Input: part model. Units: mm. Frame: model coordinates. A direction names the side the tool comes from. Coordinates: 2 decimals unless noted, no trailing zeros. Write each loop counter-clockwise with the first axis right and the second up, starting at its lowest first coordinate (ties: lowest second). Pieces come first, ordered by that corner, then holes. Notation, with made-up numbers: (75.5, 22) - (96.5, 22) arc R24 ccw to (96.5, 54) - close; hole circle Ø1 at (79, 14.25). An arc over 180 degrees is marked (long way). Put each result on its own line as item: value. Start each with the question number.
1. Line query: line 1 (Z direction, x = 0.5, y = 54); line 2 (Y direction, x = 5.5, z = 31.5); line 3 (Y direction, x = -42, z = 17). Output: solid intervals per line, ascending.
2. Cut plane D-D, the plane z = 22.5. Return loops of the section in (x, y), and give its area (3 significant figures).
3. Access query for faces 1 (the flat face through (-25.67, -70.96, 19.14)), 2 (the flat face through (31.75, -16, 16)), 3 (the flat face through (-9, 0, 25.4)), 4 (the flat face through (-6.35, 62, 38)). Directions: +Z, -Z, +X, -X, +Y, -Y. A direction counts if a zero-diameter tool reaches every point of the face in a straight line with its end or side. Return the directions, or none.
4. Pull-direction query (Y, two-part tool) for faces 5 (the cylindrical face through (-5.728, -79.117, 4.539)), 6 (the flat face through (8.733, 71.285, 21.785)), 7 (the flat face through (-40.73, -16.73, 19.14)); classes: released by +Y, released by -Y, zero draft, split by the parting line, or undercut.
5. Cut plane A-A, the plane z = 30. Return loops of the section in (x, y), and give its area (3 significant figures).
6. Pin query (flat end, axial travel): pin 1 (12 mm diameter, centred on y = -2.5, z = 30, fed in from +X); pin 2 (2 mm diameter, centred on x = 29, y = -61, fed in from +Z); pin 3 (6 mm diameter, centred on x = 26, z = 26, fed in from +Y). Return the tip coordinate at first contact, or that it passes through.
from build123d import *

# Parameters (mm, degrees)
F0_W        = 88.9
F0_H        = 165.1
F1_DEPTH    = 6.35
F2_DEPTH    = 25.4
F3_DEPTH    = 50.8
F4_R        = 6.34999
F5_C1_SIZE2 = 12.7
F5_C1_SIZE  = 7.3323484187
F5_C2_SIZE2 = 12.7
F5_C2_SIZE  = 7.3323484187
F5_C3_SIZE2 = 12.7
F5_C3_SIZE  = 7.3323484187
F5_C4_SIZE2 = 12.7
F5_C4_SIZE  = 7.3323484187
F5_C5_SIZE2 = 7.3323484187
F5_C5_SIZE  = 12.7
F5_C6_SIZE2 = 7.3323484187
F5_C6_SIZE  = 12.7
F5_C7_SIZE2 = 12.7
F5_C7_SIZE  = 7.3323484187
F5_C8_SIZE2 = 7.3323484187
F5_C8_SIZE  = 12.7


# Not quite as in the source:
# - a fillet or chamfer is up to 0.001 mm smaller than in the source, because OpenCascade refuses the exact size


with BuildPart() as f1:
    # F0 (on Top) → F1 (new body)
    with BuildSketch(Plane.XY):
        with Locations((-6.35, 1.5239301443)):
            Rectangle(F0_W, F0_H)
        Polygon((-44.45, 39.6239301443), (-44.45, 77.7239301443), (-6.35, 77.7239301443), (31.75, 77.7239301443), (31.75, -36.5760698557), (31.75, -74.6760698557), (-6.35, -74.6760698557), (-44.45, -74.6760698557), align=None, mode=Mode.SUBTRACT)
        with BuildLine():
            Line((31.75, 77.7239301443), (-6.35, 77.7239301443))
            Line((-6.35, 77.7239301443), (-6.35, 45.9739301443))
            ThreePointArc((-6.35, 45.9739301443), (-8.2098719395, 41.4838020838), (-12.7, 39.6239301443))
            Line((-12.7, 39.6239301443), (-44.45, 39.6239301443))
            Line((-44.45, 39.6239301443), (-44.45, -74.6760698557))
            Line((-44.45, -74.6760698557), (-6.35, -74.6760698557))
            Line((-6.35, -74.6760698557), (-6.35, -42.9260698557))
            ThreePointArc((-6.35, -42.9260698557), (-4.4901280605, -38.4359417952), (0, -36.5760698557))
            Line((0, -36.5760698557), (31.75, -36.5760698557))
            Line((31.75, -36.5760698557), (31.75, 77.7239301443))
        make_face()
        with BuildLine():
            Line((-6.35, 77.7239301443), (-44.45, 77.7239301443))
            Line((-44.45, 77.7239301443), (-44.45, 39.6239301443))
            Line((-44.45, 39.6239301443), (-12.7, 39.6239301443))
            ThreePointArc((-12.7, 39.6239301443), (-8.2098719395, 41.4838020838), (-6.35, 45.9739301443))
            Line((-6.35, 45.9739301443), (-6.35, 77.7239301443))
        make_face()
        with BuildLine():
            Line((31.75, -74.6760698557), (31.75, -36.5760698557))
            Line((31.75, -36.5760698557), (0, -36.5760698557))
            ThreePointArc((0, -36.5760698557), (-4.4901280605, -38.4359417952), (-6.35, -42.9260698557))
            Line((-6.35, -42.9260698557), (-6.35, -74.6760698557))
            Line((-6.35, -74.6760698557), (31.75, -74.6760698557))
        make_face()
    extrude(amount=F1_DEPTH)

    # F0 (on Top) → F2 (join)
    with BuildSketch(Plane.XY):
        with BuildLine():
            Line((31.75, 77.7239301443), (-6.35, 77.7239301443))
            Line((-6.35, 77.7239301443), (-6.35, 45.9739301443))
            ThreePointArc((-6.35, 45.9739301443), (-8.2098719395, 41.4838020838), (-12.7, 39.6239301443))
            Line((-12.7, 39.6239301443), (-44.45, 39.6239301443))
            Line((-44.45, 39.6239301443), (-44.45, -74.6760698557))
            Line((-44.45, -74.6760698557), (-6.35, -74.6760698557))
            Line((-6.35, -74.6760698557), (-6.35, -42.9260698557))
            ThreePointArc((-6.35, -42.9260698557), (-4.4901280605, -38.4359417952), (0, -36.5760698557))
            Line((0, -36.5760698557), (31.75, -36.5760698557))
            Line((31.75, -36.5760698557), (31.75, 77.7239301443))
        make_face()
    extrude(amount=F2_DEPTH)

    # F0 (on Top) → F3 (join)
    with BuildSketch(Plane.XY):
        with BuildLine():
            Line((-6.35, 77.7239301443), (-44.45, 77.7239301443))
            Line((-44.45, 77.7239301443), (-44.45, 39.6239301443))
            Line((-44.45, 39.6239301443), (-12.7, 39.6239301443))
            ThreePointArc((-12.7, 39.6239301443), (-8.2098719395, 41.4838020838), (-6.35, 45.9739301443))
            Line((-6.35, 45.9739301443), (-6.35, 77.7239301443))
        make_face()
        with BuildLine():
            Line((31.75, -74.6760698557), (31.75, -36.5760698557))
            Line((31.75, -36.5760698557), (0, -36.5760698557))
            ThreePointArc((0, -36.5760698557), (-4.4901280605, -38.4359417952), (-6.35, -42.9260698557))
            Line((-6.35, -42.9260698557), (-6.35, -74.6760698557))
            Line((-6.35, -74.6760698557), (31.75, -74.6760698557))
        make_face()
    extrude(amount=F3_DEPTH)

    # F4 (radius 6.35 in the source; OpenCascade refuses exactly that, so slightly less here)
    f4_edges = [f1.edges().sort_by_distance(p)[0] for p in [
        (38.1, 1.52393, 6.35),
        (-6.35, -81.02607, 6.35),
        (-6.35, 84.07393, 6.35),
        (-50.8, 1.52393, 6.35),
    ]]
    fillet(f4_edges, radius=F4_R)

    # F5: chamfer of 12.7 x 7.3323484187 on 8 edges, made by hand

    # F5_c1
    f5_c1_edges = [f1.edges().sort_by_distance(p)[0] for p in [
        (12.7, 77.7239301443, 25.4),
    ]]
    f5_c1_side = f1.faces().sort_by_distance((12.7, 77.7239301443, 25.2533530316))[0]
    chamfer(f5_c1_edges, length=F5_C1_SIZE, length2=F5_C1_SIZE2, reference=f5_c1_side)

    # F5_c2
    f5_c2_edges = [f1.edges().sort_by_distance(p)[0] for p in [
        (-25.4, 77.7239301443, 50.8),
    ]]
    f5_c2_side = f1.faces().sort_by_distance((-25.4, 77.7239301443, 50.6533530316))[0]
    chamfer(f5_c2_edges, length=F5_C2_SIZE, length2=F5_C2_SIZE2, reference=f5_c2_side)

    # F5_c3
    f5_c3_edges = [f1.edges().sort_by_distance(p)[0] for p in [
        (31.75, -55.6260698557, 50.8),
    ]]
    f5_c3_side = f1.faces().sort_by_distance((31.75, -55.6260698557, 50.6533530316))[0]
    chamfer(f5_c3_edges, length=F5_C3_SIZE, length2=F5_C3_SIZE2, reference=f5_c3_side)

    # F5_c4
    f5_c4_edges = [f1.edges().sort_by_distance(p)[0] for p in [
        (31.75, 14.2239301443, 25.4),
    ]]
    f5_c4_side = f1.faces().sort_by_distance((31.75, 14.2239301443, 25.2533530316))[0]
    chamfer(f5_c4_edges, length=F5_C4_SIZE, length2=F5_C4_SIZE2, reference=f5_c4_side)

    # F5_c5
    f5_c5_edges = [f1.edges().sort_by_distance(p)[0] for p in [
        (-25.4, -74.6760698557, 25.4),
    ]]
    f5_c5_side = f1.faces().sort_by_distance((-25.4, -74.6760698557, 25.2533530316))[0]
    chamfer(f5_c5_edges, length=F5_C5_SIZE, length2=F5_C5_SIZE2, reference=f5_c5_side)

    # F5_c6
    f5_c6_edges = [f1.edges().sort_by_distance(p)[0] for p in [
        (6.35, -74.6760698557, 50.8),
    ]]
    f5_c6_side = f1.faces().sort_by_distance((6.35, -74.6760698557, 50.6533530316))[0]
    chamfer(f5_c6_edges, length=F5_C6_SIZE, length2=F5_C6_SIZE2, reference=f5_c6_side)

    # F5_c7
    f5_c7_edges = [f1.edges().sort_by_distance(p)[0] for p in [
        (-44.45, 52.3239301443, 50.8),
    ]]
    f5_c7_side = f1.faces().sort_by_distance((-44.45, 52.3239301443, 50.6533530316))[0]
    chamfer(f5_c7_edges, length=F5_C7_SIZE, length2=F5_C7_SIZE2, reference=f5_c7_side)

    # F5_c8
    f5_c8_edges = [f1.edges().sort_by_distance(p)[0] for p in [
        (-44.45, -13.8598956463, 25.4),
    ]]
    f5_c8_side = f1.faces().sort_by_distance((-44.45, -13.8598956463, 25.2533530316))[0]
    chamfer(f5_c8_edges, length=F5_C8_SIZE, length2=F5_C8_SIZE2, reference=f5_c8_side)


solid = f1.part
Report:
1. line 1: z = 0 to 25.4
1. line 2: y = -74.68 to -36.58
1. line 3: y = 39.62 to 77.72
2. outline: (-44.45, 39.62) - (-38.79, 39.62) - (-38.79, -69.02) - (-6.35, -69.02) - (-6.35, -74.68) - (31.75, -74.68) - (31.75, -36.58) - (24.07, -36.58) - (24.07, 70.05) - (-6.35, 70.05) - (-6.35, 77.72) - (-44.45, 77.72) - close
2. area: 9,670 mm^2
3. face 1: +Z, -X, -Y
3. face 2: +Z, +X, +Y, -Y
3. face 3: +Z
3. face 4: +Z, +X, +Y
4. face 5: released by -Y
4. face 6: released by +Y
4. face 7: zero draft
5. outline: (-44.45, 39.62) - (-12.7, 39.62) arc R6.35 ccw to (-6.35, 45.97) - (-6.35, 77.72) - (-44.45, 77.72) - close; (-6.35, -74.68) - (31.75, -74.68) - (31.75, -36.58) - (0, -36.58) arc R6.35 ccw to (-6.35, -42.93) - close
5. area: 2,890 mm^2
6. pin 1: stops at x = 21.47
6. pin 2: stops at z = 45.63
6. pin 3: stops at y = -36.58
